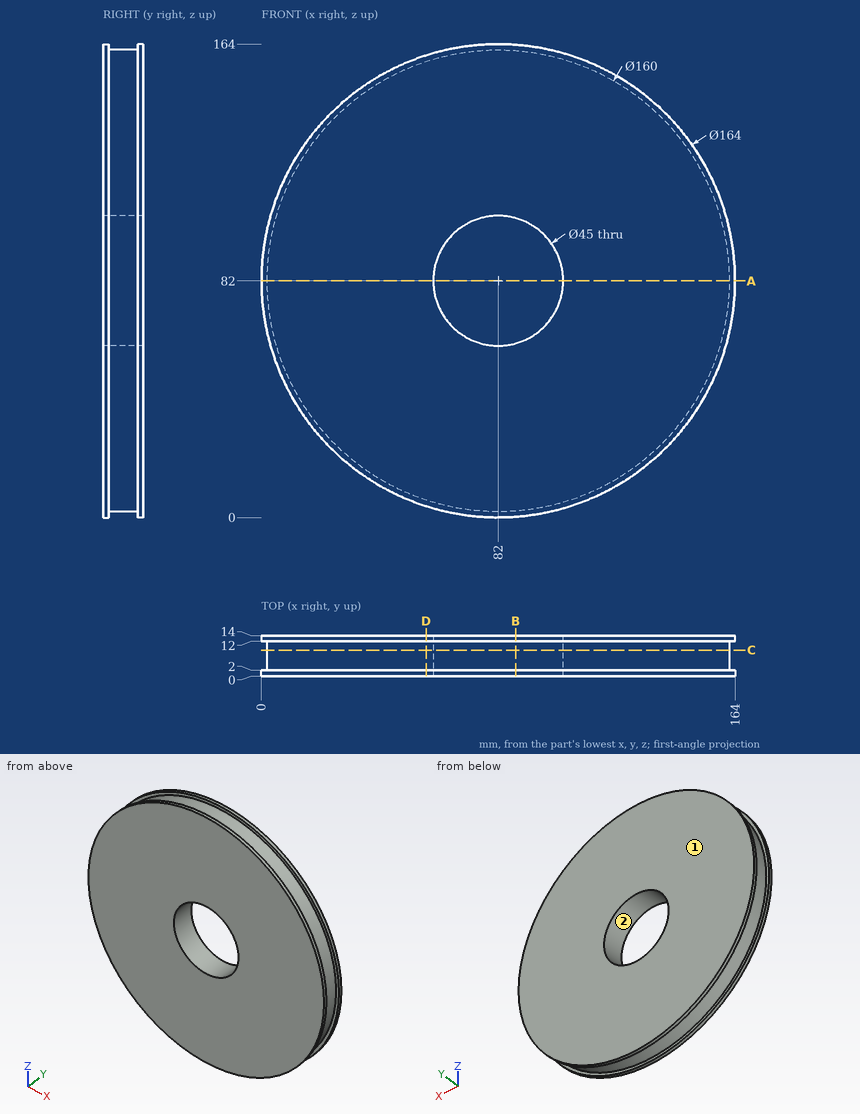
Answer from the drawing. Dimensions are ordinates in mm from the lowest x, y and z of the part. Round coordinates to 2 decimals unless told otherwise and drop trailing zeros. Order: outer loops, then holes, each group sorted by start corner. A loop starts at its lowest first (then second) coordinate and runs counter-clockwise, first axis right, second up. Notation, with made-up numbers: (60, -15.75) -> (95, -15.75) arc R13 cw to (95, 4.25) -> close; hole circle Ø11 at (-3.75, -1.5). An arc over 180 degrees is marked (long way). Answer as CSV lines item,"result".
Q1. A cutting plane is placed at B-B on x = 88. Determine the outline of the cut face in (y, z), plus the area to 3 significant figures.
Computed values:
outline,"(0, 0.22) -> (2, 0.22) -> (2, 2.23) -> (12, 2.23) -> (12, 0.22) -> (14, 0.22) -> (14, 60.31) -> (0, 60.31) -> close; (0, 103.69) -> (14, 103.69) -> (14, 163.78) -> (12, 163.78) -> (12, 161.77) -> (2, 161.77) -> (2, 163.78) -> (0, 163.78) -> close"
area,"1,640 mm^2"
Q2. Consider line 1 (Z direction, x = 82, y = 6.5); line 2 (Z direction, x = 95, y = 1.5). Determine where each line is inside the solid, lowest interval first. Write a range as from..to.
Computed values:
line 1,"z = 2..59.5, 104.5..162"
line 2,"z = 1.04..63.64, 100.36..162.96"
Q3. Given pin 1 (8 mm diameter, centred on x = 84, y = 7, fed in from +Z); pin 2 (3 mm diameter, centred on x = 18, y = 10, fed in from +Z); pin 3 (2 mm diameter, centred on x = 118.5, y = 3.5, fed in from +Z), each flat-ended and moving along its own axis, determine where each tip first touches the part or whether it passes through.
Computed values:
pin 1,"stops at z = 162"
pin 2,"stops at z = 131.94"
pin 3,"stops at z = 153.69"
Q4. A cutting plane is placed at C-C on y = 9. Determine the outline of the cut face in (x, z), plus the area to 3 significant figures.
Computed values:
outline,"circle Ø160 at (82, 82); hole circle Ø45 at (82, 82)"
area,"18,500 mm^2"
Q5. A cutting plane is placed at A-A on z = 82. Determine the outline of the cut face in (x, y), plus the area to 3 significant figures.
Computed values:
outline,"(0, 0) -> (59.5, 0) -> (59.5, 14) -> (0, 14) -> (0, 12) -> (2, 12) -> (2, 2) -> (0, 2) -> close; (104.5, 0) -> (164, 0) -> (164, 2) -> (162, 2) -> (162, 12) -> (164, 12) -> (164, 14) -> (104.5, 14) -> close"
area,"1,630 mm^2"
Q6. For a pull along Z with two mould halves and no side action, classify the marked faces 1 and 2 as +Z half, -Z half, draft (parallel to the pull), parting line (faces both ways), or undercut.
Computed values:
face 1,"draft"
face 2,"undercut"
Q7. A cutting plane is placed at D-D on x = 57. Determine the outline of the cut face in (y, z), plus the area to 3 significant figures.
Computed values:
outline,"(0, 3.9) -> (2, 3.9) -> (2, 6.01) -> (12, 6.01) -> (12, 3.9) -> (14, 3.9) -> (14, 160.1) -> (12, 160.1) -> (12, 157.99) -> (2, 157.99) -> (2, 160.1) -> (0, 160.1) -> close"
area,"2,140 mm^2"
